Can you work these out from the drawing? Everything is in mm from the part's minimum corner. A direction names the side the tool comes from. Give positions to 0.01 mm unless a question says otherwise; leave off trailing zeros. Loops run counter-clockwise (first coordinate to the right, second up) from the corner with the lowest first, then second, coordinate; pieces in that order, holes last. Notation, with made-up numbers: (21.25, 79.25) -> (56.25, 79.25) arc R29 cw to (56.25, 99.25) -> close; hole circle Ø6 at (-5.75, -26.5). An arc over 180 degrees is marked (long way). Return JSON: item names as keys, results as strings. Group by question number.
Q1. Suppose I cut it at D-D, the plane y = 9. Please give me the cut outline in (x, z).
Q2. Which directions (+Z, -Z, +X, -X, +Y, -Y) give clear straight access to the entire face, cutting with the end or side of a thin tool? Please do the marked faces 1, 2, 3 and 4.
Q3. Suppose I cut it at A-A, the plane y = 31. Please give me the cut outline in (x, z).
Q4. Will these pins go through, and if not, where does the flat tip stop? pin 1 (10.5 mm diameter, centred on y = 30, z = 17, fed in from -X); pin 2 (1.5 mm diameter, centred on y = 26.5, z = 6.5, fed in from -X); pin 3 (22 mm diameter, centred on x = 11, y = 13.5, fed in from +Z); pin 4 (17.5 mm diameter, centred on x = 44, z = 33, fed in from -Y).
Q5. Suppose I cut it at C-C, the plane z = 33. Please give me the cut outline in (x, y), and give its area (3 significant figures).
Q6. Suppose I cut it at B-B, the plane x = 8. Please give me the cut outline in (y, z), and give its area (3 significant figures).
Q7. I need wall thicknesses on line 1 along X through (y, z) = (27, 33); line 2 along Y through (x, z) = (13, 9); line 3 along Y through (x, z) = (8, 3). Which ranges of each line are inside material? Lowest first, please. Write a range as [from, to].
Q8. Thinking about a two-plate mould opening in X: for the marked faces 5, 6 and 7, which applies, pulls with the +X half, pulls with the -X half, needs draft (parallel to the pull), parting line crosses it, or undercut?
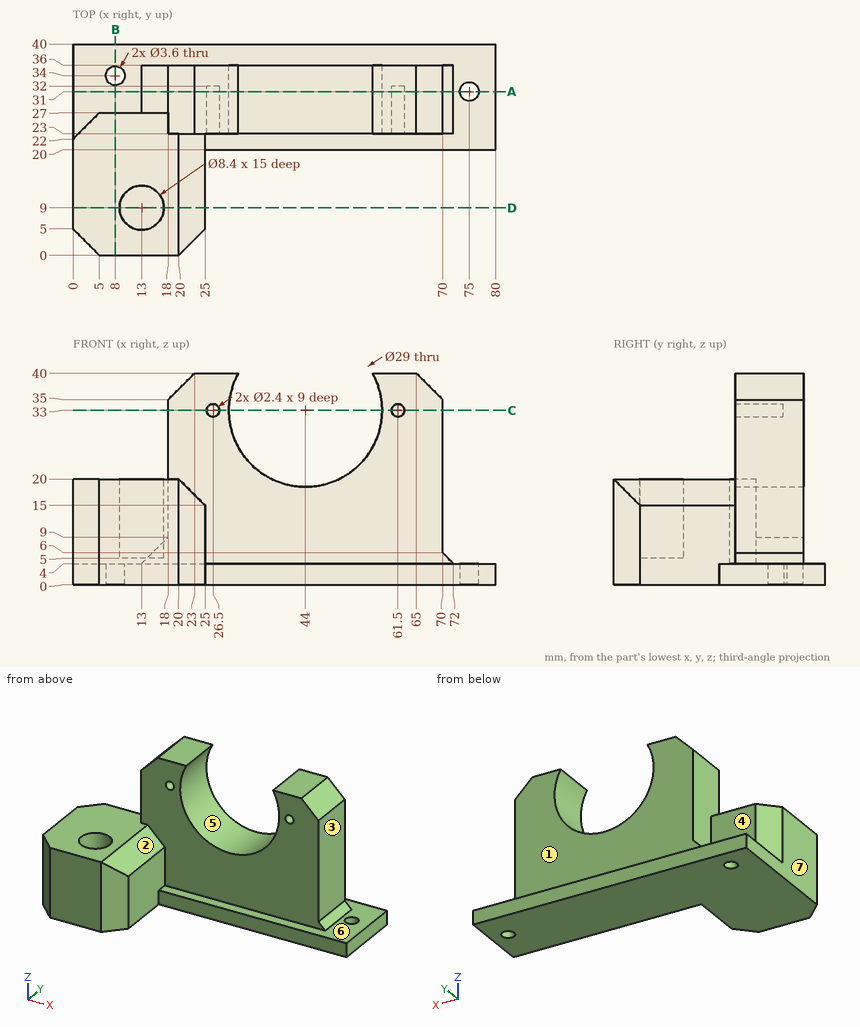
Ans:
{
 "1": {"outline": "(0, 0) -> (25, 0) -> (25, 15) -> (20, 20) -> (17.2, 20) -> (17.2, 5) -> (8.8, 5) -> (8.8, 20) -> (0, 20) -> close"},
 "2": {"face 1": "+Z, +X, -X, +Y", "face 2": "+Z, +X, -Y", "face 3": "+Z, +X, +Y, -Y", "face 4": "+Z, -X, +Y"},
 "3": {"outline": "(0, 0) -> (73.2, 0) -> (73.2, 4) -> (72, 4) -> (70, 6) -> (70, 35) -> (65, 40) -> (56.7, 40) arc R14.5 cw (long way) to (31.3, 40) -> (23, 40) -> (18, 35) -> (18, 9) -> (13, 4) -> (0, 4) -> close; (76.8, 0) -> (80, 0) -> (80, 4) -> (76.8, 4) -> close; hole circle Ø2.4 at (26.5, 33); hole circle Ø2.4 at (61.5, 33)"},
 "4": {"pin 1": "stops at x = 2.75", "pin 2": "stops at x = 3.75", "pin 3": "stops at z = 20", "pin 4": "passes through"},
 "5": {"outline": "(18, 23) -> (25.3, 23) -> (25.3, 32) -> (27.7, 32) -> (27.7, 23) -> (29.5, 23) -> (29.5, 36) -> (18, 36) -> close; (58.5, 23) -> (60.3, 23) -> (60.3, 32) -> (62.7, 32) -> (62.7, 23) -> (70, 23) -> (70, 36) -> (58.5, 36) -> close", "area": "256 mm^2"},
 "6": {"outline": "(0, 0) -> (32.2, 0) -> (32.2, 4) -> (27, 4) -> (27, 20) -> (0, 20) -> close; (35.8, 0) -> (40, 0) -> (40, 4) -> (35.8, 4) -> close", "area": "578 mm^2"},
 "7": {"line 1": "x = [18, 25.3], [27.7, 29.5], [58.5, 60.3], [62.7, 70]", "line 2": "y = [0, 4.8], [13.2, 27]", "line 3": "y = [0, 32.2], [35.8, 40]"},
 "8": {"face 5": "undercut", "face 6": "needs draft", "face 7": "pulls with the -X half"}
}
